Design review of the part built by this model. Coordinates are the model's own, in mm. Round coordinates to 2 decimals unless told otherwise and drop trailing zeros. Order: outer loops, then holes, each group sorted by start corner. A loop starts at its lowest first (then second) coordinate and runs counter-clockwise, first axis right, second up. Notation, with made-up numbers: M 66,81 L 86,81 A26 ccw 86,104 Z; hole C 4.5,15.5 d2. An arc over 180 degrees is marked long. Write each question's results on one line, items separated by ' | '. Start each with the question number.
Item 1: Clearance check with flat-ended pins moving along their axes: pin 1 (8 mm diameter, centred on y = 6.5, z = 93.5, fed in from -X); pin 2 (3 mm diameter, centred on y = 5, z = 106.5, fed in from -X); pin 3 (2 mm diameter, centred on y = 7, z = 32, fed in from +X). State where each tip first meets the part, or that it passes through.
Item 2: Take a section at C-C, the plane z = 10.5. Write out the cut boundary in (x, y).
Item 3: Take a section at B-B, the plane y = 4.5. Write out the cut boundary in (x, z).
Item 4: Take a section at D-D, the plane y = -7.75. Write out the cut boundary in (x, z), plus the area to 3 significant figures.
Item 5: Take a section at A-A, the plane x = 0. Write out the cut boundary in (y, z), plus the area to 3 significant figures.
Item 6: Wall thickness on line 1 (X direction, y = 6, z = 55.5); line 2 (Z direction, x = 1.75, y = 8.5); line 3 (X direction, y = -8, z = 57.5): over which ranges is each line inside the solid? List them lowest first. Write a range as [from, to].
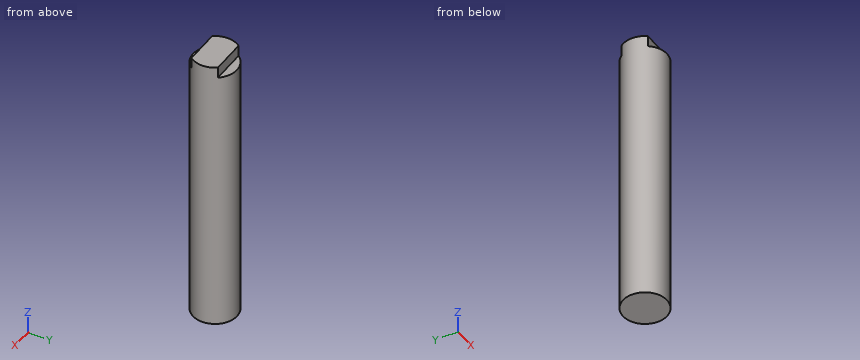
Autodesk Inventor part; units mm, degrees
ref_plane "YZ Plane" through (0, 0, 0) normal (1, 0, 0) x (0, 1, 0)
ref_plane "XZ Plane" through (0, 0, 0) normal (0, 1, 0) x (-1, 0, 0)
ref_plane "XY Plane" through (0, 0, 0) normal (0, 0, 1) x (1, 0, 0)
sketch "Эскиз1" plane through (0, 0, 0) normal (0, 0, 1) x (1, 0, 0)
  circle A0 centre (0, 0) radius 10
  dimension "d0" = 20
extrude "Выдавливание1" add sketch "Эскиз1" along normal blind 128
sketch "Эскиз2" plane through (0, 0, 128) normal (0, 0, 1) x (1, 0, 0)
  circle A0 centre (0, 0) radius 10
  line L0 (8, 6) -> (-8, 6)
  line L1 (-8, -6) -> (8, -6)
  dimension "d3" = 12
extrude "Выдавливание2" cut sketch "Эскиз2" against normal blind 5 contours L0 A0 | A0 L1
equation "\"d0\" = d_main_shaft"
equation "\"d3\" = width_flattened_surface"
equation "\"d_main_shaft\" = 20"
equation "\"tolerance_plazma\" = 0.1"
equation "\"thickness_steel\" = 3"
equation "\"d_main_screw_holes\" = 6.1"
equation "\"thickness_profile_tibea\" = 3"
equation "\"thickness_profile_femur\" = 3"
equation "\"width_flattened_surface\" = 12"
equation "\"width_shaft_shift\" = 35"
equation "\"hight_shaft_shift\" = 37"
properties part number "shaft_tibea" material "Сталь 09Г2С"
Results list:
1) pin 1: x = -9.68 | pin 2: x = -9.37 | pin 3: x = 8
2) outline: C 0,0 d20
3) outline: M -8.93,0 L 8.93,0 L 8.93,128 L -8.93,128 Z
4) outline: M -6.32,0 L 6.32,0 L 6.32,123 L -6.32,123 Z | area: 1,550 mm²
5) outline: M -10,0 L 10,0 L 10,123 L 6,123 L 6,128 L -6,128 L -6,123 L -10,123 Z | area: 2,520 mm²
6) line 1: [-8, 8] | line 2: [0, 123] | line 3: [-6, 6]
